from build123d import *

# Parameters (mm, degrees)
SKETCH_1_R      = 1.5
SKETCH_1_R_2    = 2
EXTRUDE_1_DEPTH = 6


with BuildPart() as part:
    # 草图1 → 凸台-拉伸1 (new body)
    with BuildSketch(Plane.XY):
        with BuildLine():
            Line((0, 110.847244413), (30, 110.847244413))
            Line((30, 110.847244413), (23.741384574, 117.105859839))
            ThreePointArc((23.741384574, 117.105859839), (23.229244404, 120.664151209), (26.498673071, 122.158996089))
            ThreePointArc((26.498673071, 122.158996089), (87.76795333, 89.00441769), (121.776362518, 28.20492035))
            ThreePointArc((121.776362518, 28.20492035), (120.309085428, 24.90465706), (116.732409474, 25.406681918))
            Line((116.732409474, 25.406681918), (110.847244413, 31.291846979))
            Line((110.847244413, 31.291846979), (110.847244413, 0))
            Line((110.847244413, 0), (110.847244413, -30))
            Line((110.847244413, -30), (117.105859839, -23.741384574))
            ThreePointArc((117.105859839, -23.741384574), (120.664151209, -23.229244404), (122.158996089, -26.498673071))
            ThreePointArc((122.158996089, -26.498673071), (89.29937265, -87.467834341), (29.024164684, -121.583707233))
            ThreePointArc((29.024164684, -121.583707233), (27.627313844, -121.582823674), (26.382281192, -120.949509578))
            ThreePointArc((26.382281192, -120.949509578), (0, -111.236531221), (-26.382281192, -120.949509578))
            ThreePointArc((-26.382281192, -120.949509578), (-27.627313844, -121.582823674), (-29.024164684, -121.583707233))
            ThreePointArc((-29.024164684, -121.583707233), (-88.685394575, -88.090299063), (-121.776362518, -28.20492035))
            ThreePointArc((-121.776362518, -28.20492035), (-120.309085428, -24.90465706), (-116.732409474, -25.406681918))
            Line((-116.732409474, -25.406681918), (-110.847244413, -31.291846979))
            Line((-110.847244413, -31.291846979), (-110.847244413, 0))
            Line((-110.847244413, 0), (-110.847244413, 30))
            Line((-110.847244413, 30), (-117.105859839, 23.741384574))
            ThreePointArc((-117.105859839, 23.741384574), (-120.664151209, 23.229244404), (-122.158996089, 26.498673071))
            ThreePointArc((-122.158996089, 26.498673071), (-89.00441769, 87.76795333), (-28.20492035, 121.776362518))
            ThreePointArc((-28.20492035, 121.776362518), (-24.90465706, 120.309085428), (-25.406681918, 116.732409474))
            Line((-25.406681918, 116.732409474), (-31.291846979, 110.847244413))
            Line((-31.291846979, 110.847244413), (0, 110.847244413))
        make_face()
        with Locations((27.5, 17.5)):
            Circle(SKETCH_1_R, mode=Mode.SUBTRACT)
        with Locations((35, 35)):
            Circle(SKETCH_1_R_2, mode=Mode.SUBTRACT)
        with Locations((-35, 35)):
            Circle(SKETCH_1_R_2, mode=Mode.SUBTRACT)
        with Locations((-35, -35)):
            Circle(SKETCH_1_R_2, mode=Mode.SUBTRACT)
        with Locations((35, -35)):
            Circle(SKETCH_1_R_2, mode=Mode.SUBTRACT)
        with Locations((-27.5, 17.5)):
            Circle(SKETCH_1_R, mode=Mode.SUBTRACT)
        with Locations((27.5, -17.5)):
            Circle(SKETCH_1_R, mode=Mode.SUBTRACT)
        with Locations((-27.5, -17.5)):
            Circle(SKETCH_1_R, mode=Mode.SUBTRACT)
        with Locations((32, -65.646566025)):
            Circle(SKETCH_1_R, mode=Mode.SUBTRACT)
        with Locations((-32, -65.646566025)):
            Circle(SKETCH_1_R, mode=Mode.SUBTRACT)
        with Locations((32, -107.646566025)):
            Circle(SKETCH_1_R, mode=Mode.SUBTRACT)
        with Locations((-32, -107.646566025)):
            Circle(SKETCH_1_R, mode=Mode.SUBTRACT)
        with Locations((24, 85)):
            Circle(SKETCH_1_R, mode=Mode.SUBTRACT)
        with Locations((-24, 85)):
            Circle(SKETCH_1_R, mode=Mode.SUBTRACT)
        with Locations((77.23579893, 78.323887567)):
            Circle(SKETCH_1_R, mode=Mode.SUBTRACT)
        with Locations((78.323887567, -77.23579893)):
            Circle(SKETCH_1_R, mode=Mode.SUBTRACT)
        with Locations((-77.23579893, -78.323887567)):
            Circle(SKETCH_1_R, mode=Mode.SUBTRACT)
        with Locations((-78.323887567, 77.23579893)):
            Circle(SKETCH_1_R, mode=Mode.SUBTRACT)
        with BuildLine():
            Line((72.581523243, -91.765584419), (66.377974248, -83.922372075))
            Line((66.377974248, -83.922372075), (42.940005539, -108.835453435))
            ThreePointArc((42.940005539, -108.835453435), (58.387935484, -101.389590146), (72.581523243, -91.765584419))
        make_face(mode=Mode.SUBTRACT)
        with BuildLine():
            Line((91.765584419, 72.581523243), (83.922372075, 66.377974248))
            Line((83.922372075, 66.377974248), (108.835453435, 42.940005539))
            ThreePointArc((108.835453435, 42.940005539), (101.389590146, 58.387935484), (91.765584419, 72.581523243))
        make_face(mode=Mode.SUBTRACT)
        with BuildLine():
            Line((65.197518305, 84.842699196), (41.413342405, 109.425477248))
            ThreePointArc((41.413342405, 109.425477248), (56.963918445, 102.196438272), (71.290744315, 92.77192342))
            Line((71.290744315, 92.77192342), (65.197518305, 84.842699196))
        make_face(mode=Mode.SUBTRACT)
        with BuildLine():
            Line((84.842699196, -65.197518305), (109.425477248, -41.413342405))
            ThreePointArc((109.425477248, -41.413342405), (102.196438272, -56.963918445), (92.77192342, -71.290744315))
            Line((92.77192342, -71.290744315), (84.842699196, -65.197518305))
        make_face(mode=Mode.SUBTRACT)
        with BuildLine():
            Line((-91.765584419, -72.581523243), (-83.922372075, -66.377974248))
            Line((-83.922372075, -66.377974248), (-108.835453435, -42.940005539))
            ThreePointArc((-108.835453435, -42.940005539), (-101.389590146, -58.387935484), (-91.765584419, -72.581523243))
        make_face(mode=Mode.SUBTRACT)
        with BuildLine():
            Line((-65.197518305, -84.842699196), (-41.413342405, -109.425477248))
            ThreePointArc((-41.413342405, -109.425477248), (-56.963918445, -102.196438272), (-71.290744315, -92.77192342))
            Line((-71.290744315, -92.77192342), (-65.197518305, -84.842699196))
        make_face(mode=Mode.SUBTRACT)
        with BuildLine():
            Line((-72.581523243, 91.765584419), (-66.377974248, 83.922372075))
            Line((-66.377974248, 83.922372075), (-42.940005539, 108.835453435))
            ThreePointArc((-42.940005539, 108.835453435), (-58.387935484, 101.389590146), (-72.581523243, 91.765584419))
        make_face(mode=Mode.SUBTRACT)
        with BuildLine():
            Line((-84.842699196, 65.197518305), (-109.425477248, 41.413342405))
            ThreePointArc((-109.425477248, 41.413342405), (-102.196438272, 56.963918445), (-92.77192342, 71.290744315))
            Line((-92.77192342, 71.290744315), (-84.842699196, 65.197518305))
        make_face(mode=Mode.SUBTRACT)
    extrude(amount=EXTRUDE_1_DEPTH)


solid = part.part
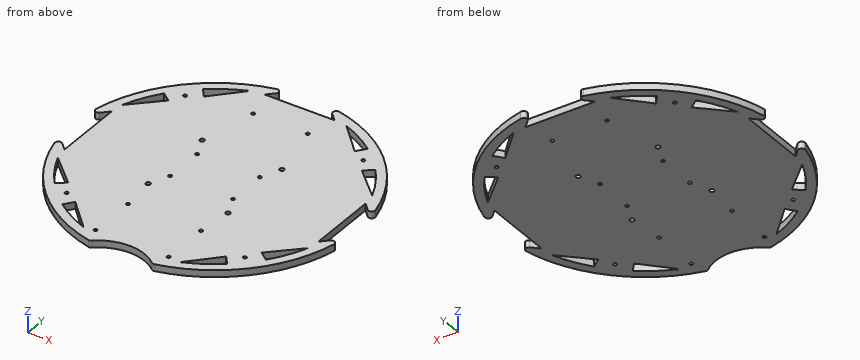
Verification items for the finished model (mm, model axes). Give positions to 0.01 mm unless a question says otherwise; leave off trailing zeros. Write each loop counter-clockwise with the first axis right and the second up, starting at its lowest first coordinate (ties: lowest second). Pieces come first, ordered by that corner, then holes.
(1) Material ranges on line 1 (Y direction, x = -35, z = 4.1); line 2 (X direction, y = 103, z = 1.5); line 3 (Y direction, x = 32, z = 1.45), recorded low to high.
(2) Cross-section at B-B (y = 51). Enter the section's corners in (x, z).
(3) Gauge pin test, flat ends, axial feed: pin 1 (3 mm diameter, centred on y = 55, z = 1, fed in from +X); pin 2 (3 mm diameter, centred on x = -52, z = 2.5, fed in from +Y); pin 3 (1 mm diameter, centred on x = -25.5, z = 1, fed in from +Y). Record the tip position at first contact, or that the pin passes through.
(4) Cross-section at D-D (x = 13). Enter the section's corners in (y, z).
(5) Cross-section at A-A (x = -99.5). Enter the section's corners in (y, z), plus the area to 3 significant figures.
(6) Cross-section at C-C (y = -4). Enter the section's corners in (x, z), plus the area to 3 significant figures.
Worked out:
1. line 1: y = -120 to -37, -33 to 33, 37 to 120
1. line 2: x = -70.82 to -55.5, -48.43 to 47.63, 55.5 to 70.82
1. line 3: y = -120.83 to -109.15, -106.15 to -67.15, -64.15 to 120.83
2. outline: (-114.12, 0) - (-105.3, 0) - (-105.3, 6) - (-114.12, 6) - close; (-99.52, 0) - (100.27, 0) - (100.27, 6) - (-99.52, 6) - close; (105.3, 0) - (114.12, 0) - (114.12, 6) - (105.3, 6) - close
3. pin 1: stops at x = 112.97
3. pin 2: stops at y = 114.34
3. pin 3: stops at y = 121.44
4. outline: (-113.37, 0) - (110.85, 0) - (110.85, 6) - (-113.37, 6) - close
5. outline: (-75.66, 0) - (-61.55, 0) - (-61.55, 6) - (-75.66, 6) - close; (-51.72, 0) - (51.02, 0) - (51.02, 6) - (-51.72, 6) - close; (61.55, 0) - (75.66, 0) - (75.66, 6) - (61.55, 6) - close
5. area: 786 mm2
6. outline: (-110.85, 0) - (110.85, 0) - (110.85, 6) - (-110.85, 6) - close
6. area: 1,330 mm2
